from build123d import *

# Parameters (mm, degrees)
SKETCH001_R   = 80
SKETCH001_R_2 = 50
PAD001_DEPTH  = 10
FILLET001_R   = 1


with BuildPart() as part:
    # Sketch001 → Pad001 (new body)
    with BuildSketch(Plane.XY):
        Circle(SKETCH001_R)
        Circle(SKETCH001_R_2, mode=Mode.SUBTRACT)
    extrude(amount=PAD001_DEPTH)

    # Fillet001
    fillet001_edges = [part.edges().sort_by_distance(p)[0] for p in [
        (-80, 0, 10),
        (-80, 0, 0),
        (-50, 0, 10),
        (-50, 0, 0),
    ]]
    fillet(fillet001_edges, radius=FILLET001_R)


with BuildPart() as part_1:
    # Body001 placement: moved
    add(part.part.moved(Location((0, 0, -59))))


solid = part_1.part
Model file for the job. Use its own axes, mm. Give positions to 0.01 mm unless a question says otherwise; leave off trailing zeros. Loops run counter-clockwise (first coordinate to the right, second up) from the corner with the lowest first, then second, coordinate; pieces in that order, holes last. Notation, with made-up numbers: (88.25, 7) - (96.25, 7) arc R28 cw to (96.25, 32) - close; hole circle Ø8 at (38, 41.25). An arc over 180 degrees is marked (long way). Use one line per item in the form item = value.
(1) Cut at C-C (z = -54.25). Give the cut face in (x, y).
Determined:
outline = circle Ø160 at (0, 0); hole circle Ø100 at (0, 0)
(2) Drop flat-ended pins along their axis: P1, Ø1, axis at y = -42, z = -57.5, coming from the +X side; P2, Ø1.5, axis at x = 3, z = -53.5, coming from the +Y side; P3, Ø6, axis at y = -16.5, z = -57, coming from the -X side. Give the stop position or say it passes through.
Determined:
P1 = 68.39
P2 = 79.97
P3 = -78.85
(3) Pull direction X, two halves, no side cores. Call faces 1 (the face through (-1, -52, -59)), 2 (the face through (47.69, 15.02, -54.06)), 3 (the face through (-17.34, -78.1, -54.06)): pulls with the +X half, pulls with the -X half, needs draft (parallel to the pull), parting line crosses it, or undercut.
Determined:
face_1 = needs draft
face_2 = undercut
face_3 = parting line crosses it
(4) Drill centre lines: L1, parallel to Y at x = 0, z = -55.75; L2, parallel to X at y = -37, z = -52.5; L3, parallel to Y at x = 25.5, z = -50. Where is each one in solid material? Low to high.
Determined:
L1 = -80 to -50, 50 to 80
L2 = -70.93 to -33.63, 33.63 to 70.93
L3 = -75.83 to -43.01, 43.01 to 75.83
(5) Cut at A-A (x = 0). Give the cut face in (y, z).
Determined:
outline = (-80, -58) arc R1 ccw to (-79, -59) - (-51, -59) arc R1 ccw to (-50, -58) - (-50, -50) arc R1 ccw to (-51, -49) - (-79, -49) arc R1 ccw to (-80, -50) - close; (50, -58) arc R1 ccw to (51, -59) - (79, -59) arc R1 ccw to (80, -58) - (80, -50) arc R1 ccw to (79, -49) - (51, -49) arc R1 ccw to (50, -50) - close
